Part model, mm, in its own coordinate system. Coordinates: 2 decimals unless noted, no trailing zeros. Loops run counter-clockwise (first coordinate to the right, second up) from the corner with the lowest first, then second, coordinate; pieces in that order, holes last. Notation, with made-up numbers: (47.25, 41) - (77.25, 41) arc R18 cw to (77.25, 52) - close; hole circle Ø6 at (65.25, 37.5). An arc over 180 degrees is marked (long way). Use a Markdown table: item, result. Add a question column.
1. Band-saw the part on A-A, the plane z = -1.7. Give the cut face in (x, y), plus the area to 3 significant figures.
2. Band-saw the part on C-C, the plane y = 14.8. Give the cut face in (x, z), plus the area to 3 significant figures.
3. Wall check: probe 1 along X at (y, z) = (76, -2.05); probe 2 along Y at (x, z) = (-15, -1.4); probe 3 along Y at (x, z) = (-16, 1.8). Give the ranges that are in metal, low to high. Write a range as [from, to].
4. Band-saw the part on B-B, the plane x = -15. Give the cut face in (y, z), plus the area to 3 significant figures.
5. Drop a flat-ended pin along its axis: pin 1 (1 mm diameter, centred on y = 80.5, z = -2, fed in from -X). Give the stop position or say it passes through.
6. Band-saw the part on D-D, the plane y = 83. Give the cut face in (x, z), plus the area to 3 significant figures.
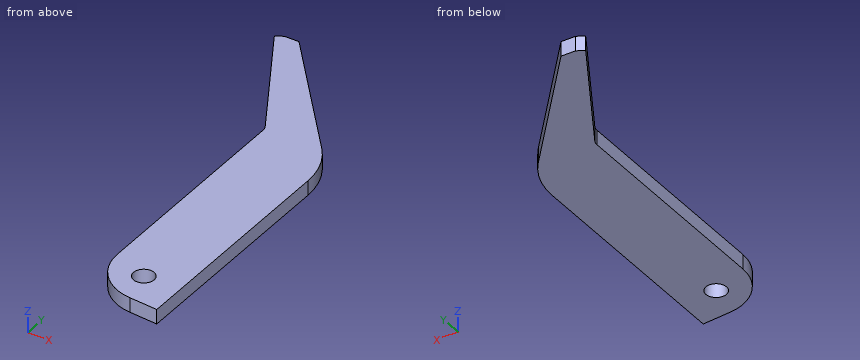
from build123d import *

# Parameters (mm, degrees)
SKETCH1_R      = 4.25
EXTRUDE1_DEPTH = 3
FILLET1_R      = 20


with BuildPart() as part:
    # Sketch1 → Extrude1 (new, symmetric)
    with BuildSketch(Plane.XY):
        with BuildLine():
            Line((0, 0), (0, 95))
            ThreePointArc((0, 95), (-1.809221376, 105.2606043), (-7.018666706, 114.283628291))
            Line((-7.018666706, 114.283628291), (-49.574755502, 165))
            Line((-49.574755502, 165), (-55.574755502, 165))
            Line((-55.574755502, 165), (-58.574755502, 163.267949192))
            Line((-58.574755502, 163.267949192), (-30.669872981, 114.935274886))
            ThreePointArc((-30.669872981, 114.935274886), (-30.170370869, 113.729370112), (-30, 112.435274886))
            Line((-30, 112.435274886), (-30, 2.624659906))
            Line((-30, 2.624659906), (0, 0))
        make_face()
        with Locations((-15, 14.8)):
            Circle(SKETCH1_R, mode=Mode.SUBTRACT)
    extrude(amount=EXTRUDE1_DEPTH, both=True)

    # Fillet1
    fillet1_edges = [part.edges().sort_by_distance(p)[0] for p in [
        (-30, 2.624659906, 0),
    ]]
    fillet(fillet1_edges, radius=FILLET1_R)


solid = part.part
Geometry check:
| question | item | result |
|---|---|---|
| 1 | outline | (-58.57, 163.27) - (-30.67, 114.94) arc R5 cw to (-30, 112.44) - (-30, 20.95) arc R20 ccw to (-11.74, 1.03) - (0, 0) - (0, 95) arc R30 ccw to (-7.02, 114.28) - (-49.57, 165) - (-55.57, 165) - close; hole circle Ø8.5 at (-15, 14.8) |
| 1 | area | 4,060 mm^2 |
| 2 | outline | (-29.03, -3) - (-19.25, -3) - (-19.25, 3) - (-29.03, 3) - close; (-10.75, -3) - (0, -3) - (0, 3) - (-10.75, 3) - close |
| 2 | area | 123 mm^2 |
| 3 | probe 1 | x = [-30, 0] |
| 3 | probe 2 | y = [1.59, 10.55], [19.05, 123.8] |
| 3 | probe 3 | y = [1.87, 10.67], [18.93, 124.99] |
| 4 | outline | (1.59, -3) - (10.55, -3) - (10.55, 3) - (1.59, 3) - close; (19.05, -3) - (123.8, -3) - (123.8, 3) - (19.05, 3) - close |
| 4 | area | 682 mm^2 |
| 5 | pin 1 | stops at x = -30 |
| 6 | outline | (-30, -3) - (0, -3) - (0, 3) - (-30, 3) - close |
| 6 | area | 180 mm^2 |
